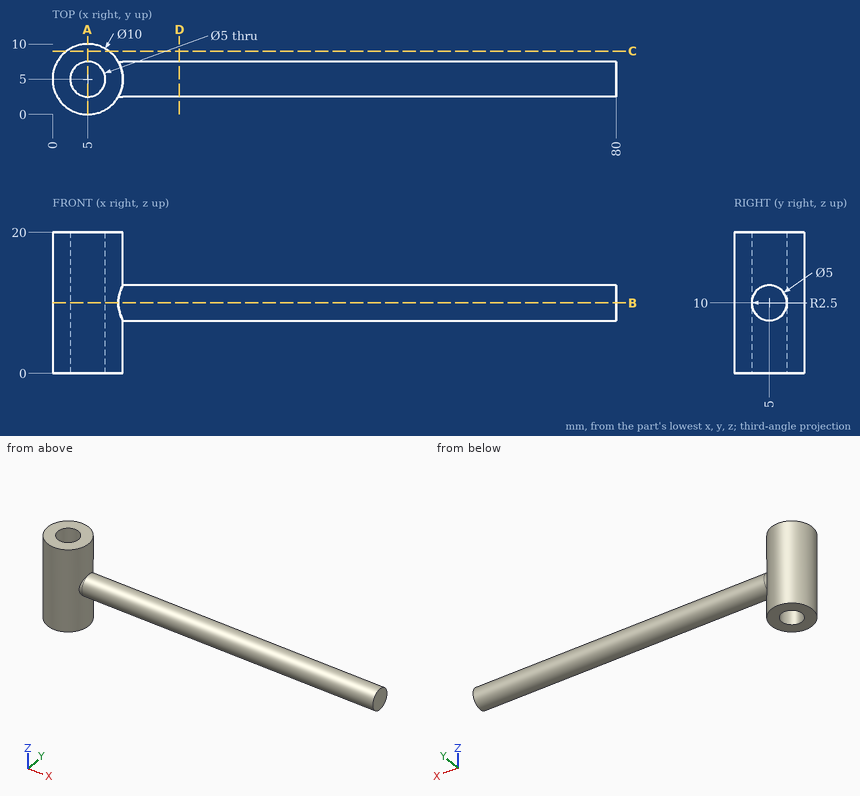
The drawing under review shows one solid part. Ordinate dimensions are in mm from its lowest x, y, z. Coordinates: 2 decimals unless noted, no trailing zeros. Order: outer loops, then holes, each group sorted by start corner. A loop starts at its lowest first (then second) coordinate and runs counter-clockwise, first axis right, second up. Notation, with made-up numbers: M 59,37 L 102,37 A17 ccw 102,65 Z; hole C 69,26.25 d2. An arc over 180 degrees is marked long. Use a Markdown table: item, result.
(1) Wall thickness on probe 1 along Y at (x, z) = (5, 16.25); probe 2 along X at (y, z) = (4.5, 9.25); probe 3 along X at (y, z) = (5.5, 14.5): over which ranges is each line inside the solid? List them lowest first.
Worked answers:
| item | result |
|---|---|
| probe 1 | y = 0 to 2.5, 7.5 to 10 |
| probe 2 | x = 0.03 to 2.55, 7.45 to 80 |
| probe 3 | x = 0.03 to 2.55, 7.45 to 9.97 |
(2) Add section D-D (x = 18). Give the boundary of the cut face in (y, z).
Worked answers:
| item | result |
|---|---|
| outline | C 5,10 d5 |
(3) For P1, Ø3, axis at x = 5, y = 5, coming from the +Z side; P2, Ø6, axis at x = 46.5, z = 13.5, coming from the -Y side; P3, Ø1.5, axis at y = 3.5, z = 15, coming from the -X side; P4, Ø10, axis at x = 50, z = 5.5, coming from the -Y side, all flat-tipped, find the tip position at first contact; note any pin that passes through.
Worked answers:
| item | result |
|---|---|
| P1 | passes through |
| P2 | stops at y = 2.55 |
| P3 | stops at x = 0.06 |
| P4 | stops at y = 2.5 |
(4) Add section B-B (z = 10). Give the boundary of the cut face in (x, y), then the cut area to 3 significant figures.
Worked answers:
| item | result |
|---|---|
| outline | M 9.33,2.5 L 80,2.5 L 80,7.5 L 9.33,7.5 A5 ccw long Z; hole C 5,5 d5 |
| area | 410 mm2 |
(5) Add section A-A (x = 5). Give the boundary of the cut face in (y, z).
Worked answers:
| item | result |
|---|---|
| outline | M 0,0 L 2.5,0 L 2.5,20 L 0,20 Z; M 7.5,0 L 10,0 L 10,20 L 7.5,20 Z |
(6) Add section C-C (y = 9). Give the boundary of the cut face in (x, z).
Worked answers:
| item | result |
|---|---|
| outline | M 2,0 L 8,0 L 8,20 L 2,20 Z |
